Read the model definition and answer for the solid it produces. Units are mm, in the model's axes. Coordinates: 2 decimals unless noted, no trailing zeros. Loops run counter-clockwise (first coordinate to the right, second up) from the corner with the lowest first, then second, coordinate; pieces in that order, holes last. Notation, with made-up numbers: (37.25, 83) -> (42.25, 83) arc R29 ccw to (42.25, 105) -> close; hole circle Ø6 at (88.5, -30.5). An arc over 180 degrees is marked (long way). Answer as a JSON object with one key per item and string values. Group by question number.
1) Section B-B, the plane x = -9.5 is taken. Give the vertices of the cut face in (y, z) (3 decimals), plus the area to 3 significant figures.
2) Flat-ended cylindrical pins translate along their axes: P1, Ø1.9, axis at x = -9.69, z = 20.8, coming from the +Y side; P2, Ø1.5, axis at x = 11, y = 2.5, coming from the +Z side (3 decimals). Find the tip coordinate at first contact, or state that the pin passes through.
3) Determine the mould class of faces 1 (the face through (26.526, 1.565, -12.923)), 2 (the face through (15.185, 1.565, -8.282)), 3 (the face through (5, 3.175, 5)) for opening direction X: released by +X, released by -X, zero draft, split by the parting line, or undercut.
4) Consider probe 1 along Z at (x, y) = (-10.5, 0.4); probe 2 along Z at (x, y) = (-10, 2.9) (3 decimals); probe 3 along X at (y, z) = (1.75, 13.5) (3 decimals). Determine where each line is inside the solid, lowest interval first. Write a range as [from, to].
5) Section A-A, the plane x = 15 is taken. Give the vertices of the cut face in (y, z) (3 decimals), plus the area to 3 significant figures.
6) Section C-C, the plane y = 1.15 is taken. Give the vertices of the cut face in (x, z) (1 decimal).
7) Section D-D, the plane z = 17.5 is taken. Give the vertices of the cut face in (x, y) (3 decimals).
from build123d import *

# Parameters (mm, degrees)
SKETCH1_R           = 1.5875
BOSS_EXTRUDE1_DEPTH = 3.175


with BuildPart() as part:
    # Sketch1 → Boss-Extrude1 (new body)
    with BuildSketch(Plane(origin=(0, 0, 0), x_dir=(1, 0, 0), z_dir=(0, 1, 0))):
        with BuildLine():
            Line((-14.452594388, -14.452594388), (14.452594388, 14.452594388))
            Line((14.452594388, 14.452594388), (24.19549194, 14.452594388))
            ThreePointArc((24.19549194, 14.452594388), (26.542145952, 12.884610306), (25.991543164, 10.116543164))
            Line((25.991543164, 10.116543164), (-10.116543164, -25.991543164))
            ThreePointArc((-10.116543164, -25.991543164), (-12.884610306, -26.542145952), (-14.452594388, -24.19549194))
            Line((-14.452594388, -24.19549194), (-14.452594388, -14.452594388))
        make_face()
        with Locations((-9.690094388, -14.452594388)):
            Circle(SKETCH1_R, mode=Mode.SUBTRACT)
        with Locations((-9.690094388, -20.802594388)):
            Circle(SKETCH1_R, mode=Mode.SUBTRACT)
        with Locations((20.802594388, 9.690094388)):
            Circle(SKETCH1_R, mode=Mode.SUBTRACT)
        with Locations((14.452594388, 9.690094388)):
            Circle(SKETCH1_R, mode=Mode.SUBTRACT)
    extrude(amount=BOSS_EXTRUDE1_DEPTH)


solid = part.part
Determined:
{
 "1": {"outline": "(0, 9.5) -> (3.175, 9.5) -> (3.175, 12.877) -> (0, 12.877) -> close; (0, 16.029) -> (3.175, 16.029) -> (3.175, 19.227) -> (0, 19.227) -> close; (0, 22.379) -> (3.175, 22.379) -> (3.175, 25.375) -> (0, 25.375) -> close", "area": "30.4 mm²"},
 "2": {"P1": "through", "P2": "z = 5.625"},
 "3": {"face 1": "released by +X", "face 2": "undercut", "face 3": "zero draft"},
 "4": {"probe 1": "[10.5, 13.09], [15.82, 19.44], [22.17, 26.31]", "probe 2": "[10, 12.896], [16.01, 19.246], [22.36, 25.875]", "probe 3": "[-13.5, -10.96], [-8.42, 2.375]"},
 "5": {"outline": "(0, -14.453) -> (3.175, -14.453) -> (3.175, -11.18) -> (0, -11.18) -> close; (0, -8.2) -> (3.175, -8.2) -> (3.175, 0.875) -> (0, 0.875) -> close", "area": "39.2 mm²"},
 "6": {"outline": "(-14.5, 14.5) -> (14.5, -14.5) -> (24.2, -14.5) arc R2.5 ccw to (26, -10.1) -> (-10.1, 26) arc R2.5 ccw to (-14.5, 24.2) -> close; hole circle Ø3.2 at (-9.7, 14.5); hole circle Ø3.2 at (-9.7, 20.8); hole circle Ø3.2 at (14.5, -9.7); hole circle Ø3.2 at (20.8, -9.7)"},
 "7": {"outline": "(-14.453, 0) -> (-1.625, 0) -> (-1.625, 3.175) -> (-14.453, 3.175) -> close"}
}
